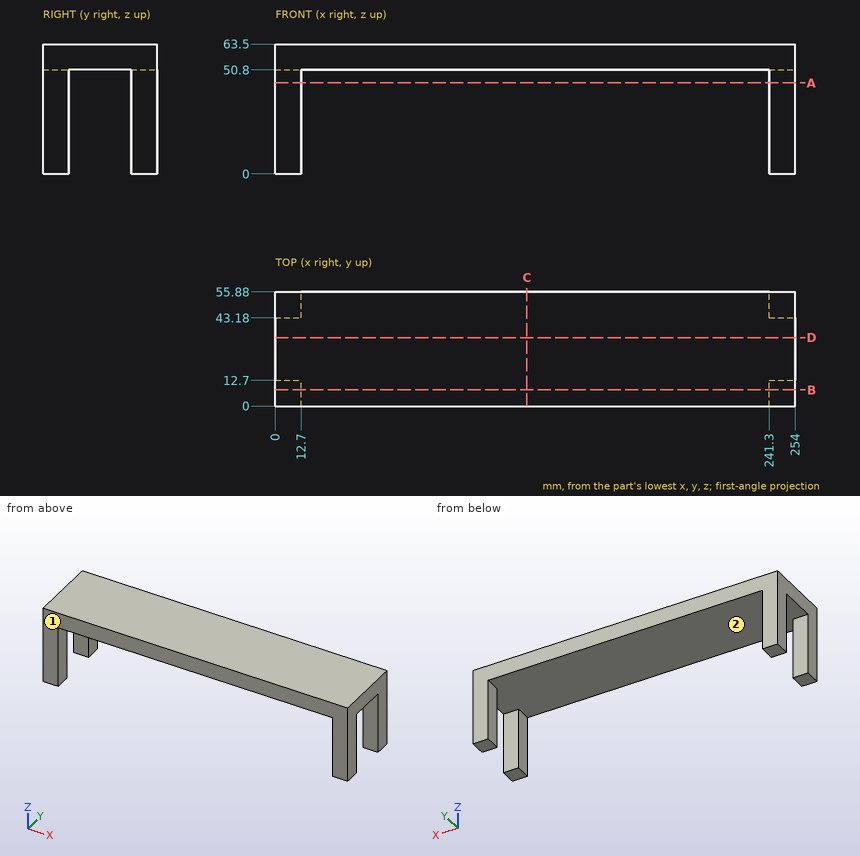
Here's the drawing with two shaded views (mm, measured from the low corner). I have some questions. Give positions to 0.01 mm unless a question says otherwise; leave off trailing zeros. Write each loop counter-clockwise with the first axis right and the second up, starting at its lowest first coordinate (ties: lowest second). Pieces come first, ordered by that corner, then holes. Notation, with made-up numbers: (-35, 25.5) -> (18, 25.5) arc R22 ccw to (18, 44.5) -> close; hole circle Ø2 at (-30.5, 64). An arc over 180 degrees is marked (long way). Use one line per item in the form item = value. Start each with the question number.
1. Imagine slicing it at D-D on y = 33.5. List the corners of the cut face in (x, z) for me.
2. Imagine slicing it at A-A on z = 44.5. List the corners of the cut face in (x, y) for me, plus the area to 3 significant figures.
3. Imagine slicing it at C-C on x = 123. List the corners of the cut face in (y, z) for me.
4. If I drill on L1, parallel to X at y = 4.5, z = 15.5; L2, parallel to Z at x = 72, y = 33.5, over which ranges is the centre line in solid material (lowest first)?
5. Imagine slicing it at B-B on y = 8. List the corners of the cut face in (x, z) for me, plus the area to 3 significant figures.
6. Will this pin go through, and if not, where does the flat tip stop? pin 1 Ø8 at (x, y) = (175.5, 26) entering from -Z.
7. Thinking about a two-plate mould opening in X: for the marked faces 1 and 2, which applies, +X half, -X half, draft (parallel to the pull), parting line (faces both ways), or undercut?
Entries:
q1.outline = (0, 50.8) -> (254, 50.8) -> (254, 63.5) -> (0, 63.5) -> close
q2.outline = (0, 0) -> (12.7, 0) -> (12.7, 12.7) -> (0, 12.7) -> close; (0, 43.18) -> (12.7, 43.18) -> (12.7, 55.88) -> (0, 55.88) -> close; (241.3, 0) -> (254, 0) -> (254, 12.7) -> (241.3, 12.7) -> close; (241.3, 43.18) -> (254, 43.18) -> (254, 55.88) -> (241.3, 55.88) -> close
q2.area = 645 mm²
q3.outline = (0, 50.8) -> (55.88, 50.8) -> (55.88, 63.5) -> (0, 63.5) -> close
q4.L1 = 0 to 12.7, 241.3 to 254
q4.L2 = 50.8 to 63.5
q5.outline = (0, 0) -> (12.7, 0) -> (12.7, 50.8) -> (241.3, 50.8) -> (241.3, 0) -> (254, 0) -> (254, 63.5) -> (0, 63.5) -> close
q5.area = 4,520 mm²
q6.pin_1 = 50.8
q7.face_1 = draft
q7.face_2 = undercut
